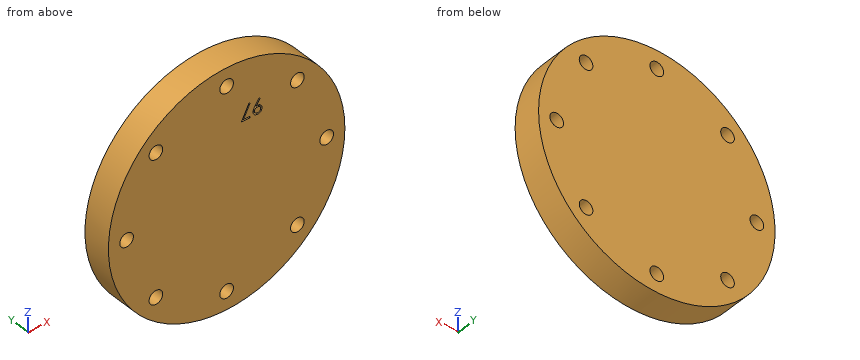
from build123d import *

# Parameters (mm, degrees)
SKETCH1_R           = 26
BOSS_EXTRUDE1_DEPTH = 6.2
SKETCH4_R           = 1.5
CUT_EXTRUDE1_DEPTH  = 13
SKETCH5_R           = 1.5
CUT_EXTRUDE2_DEPTH  = 10
CUT_EXTRUDE3_DEPTH  = 1


with BuildPart() as part:
    # Sketch1 → Boss-Extrude1 (new body)
    with BuildSketch(Plane(origin=(0, 0, 0), x_dir=(1, 0, 0), z_dir=(0, 1, 0))):
        Circle(SKETCH1_R)
    extrude(amount=BOSS_EXTRUDE1_DEPTH)

    # Sketch4 → Cut-Extrude1 (cut)
    with BuildSketch(Plane.XZ):
        with Locations((22, 0)):
            Circle(SKETCH4_R)
    extrude(amount=-CUT_EXTRUDE1_DEPTH, mode=Mode.SUBTRACT)

    # Sketch5 → Cut-Extrude2 (cut)
    with BuildSketch(Plane.XZ):
        with Locations((-22, 0)):
            Circle(SKETCH5_R)
        with Locations((0, 22)):
            Circle(SKETCH5_R)
        with Locations((0, -22)):
            Circle(SKETCH5_R)
        with Locations((-15.556349186, 15.556349186)):
            Circle(SKETCH5_R)
        with Locations((15.556349186, 15.556349186)):
            Circle(SKETCH5_R)
        with Locations((15.556349186, -15.556349186)):
            Circle(SKETCH5_R)
        with Locations((-15.556349186, -15.556349186)):
            Circle(SKETCH5_R)
    extrude(amount=-CUT_EXTRUDE2_DEPTH, mode=Mode.SUBTRACT)

    # Sketch6 → Cut-Extrude3 (cut)
    with BuildSketch(Plane(origin=(0, 0, 0), x_dir=(-1, 0, 0), z_dir=(0, -1, 0))):
        with BuildLine():
            Line((-7.133469585, -15.941578498), (-7.361163896, -15.783210108))
            Line((-7.361163896, -15.783210108), (-6.478371428, -14.492730341))
            add(Edge.make_bspline(
                [(-6.478371428, -14.492730341), (-6.534696595, -14.499618334), (-6.64560399, -14.513181177), (-6.757306933, -14.515672785), (-6.812280683, -14.516899011)],
                knots=[0, 0, 0, 0, 0.000170115, 0.000334967, 0.000334967, 0.000334967, 0.000334967], degree=3))
            add(Edge.make_bspline(
                [(-6.812280683, -14.516899011), (-6.845610969, -14.51604532), (-6.911035406, -14.5143696), (-7.007221263, -14.501087388), (-7.099646021, -14.4806312), (-7.188064651, -14.450106973), (-7.272809488, -14.412171883), (-7.353695528, -14.365130163), (-7.430613885, -14.309788742), (-7.502738465, -14.246440242), (-7.568335542, -14.176882295), (-7.626776676, -14.103262533), (-7.675346132, -14.02472576), (-7.715692748, -13.94287406), (-7.746291089, -13.856530978), (-7.768572819, -13.766679022), (-7.782290955, -13.672688461), (-7.783922991, -13.608712092), (-7.784751636, -13.576228939)],
                knots=[0, 0, 0, 0, 9.9954e-05, 0.000196201, 0.000290782, 0.000383503, 0.000476303, 0.000568919, 0.000663705, 0.000760153, 0.000856434, 0.000950205, 0.001041624, 0.001132931, 0.001223461, 0.001315861, 0.001410305, 0.001507717, 0.001507717, 0.001507717, 0.001507717], degree=3))
            add(Edge.make_bspline(
                [(-7.784751636, -13.576228939), (-7.783178256, -13.531807375), (-7.78009003, -13.444616857), (-7.755235661, -13.317223367), (-7.714359496, -13.196767002), (-7.657365183, -13.083564469), (-7.585578686, -12.979244184), (-7.499301608, -12.885256374), (-7.399058726, -12.802937828), (-7.287133608, -12.732176987), (-7.166163368, -12.675267382), (-7.039463942, -12.633321731), (-6.908006134, -12.608648581), (-6.818954033, -12.605395693), (-6.774119625, -12.603757985)],
                knots=[0, 0, 0, 0, 0.000133185, 0.000261414, 0.000387724, 0.00051373, 0.000640399, 0.00076644, 0.000895188, 0.001028407, 0.001162697, 0.001295241, 0.001427846, 0.0015623, 0.0015623, 0.0015623, 0.0015623], degree=3))
            add(Edge.make_bspline(
                [(-6.774119625, -12.603757985), (-6.730133702, -12.605418204), (-6.643221663, -12.608698641), (-6.515415207, -12.632723385), (-6.393004427, -12.673215224), (-6.276667904, -12.729171935), (-6.168954294, -12.799313044), (-6.072093379, -12.882892219), (-5.988295569, -12.979961519), (-5.917698191, -13.088173221), (-5.861028941, -13.204438982), (-5.820141941, -13.325800112), (-5.794972683, -13.451383809), (-5.791801015, -13.536468796), (-5.790200354, -13.579409027)],
                knots=[0, 0, 0, 0, 0.000131915, 0.000260652, 0.000388569, 0.000517718, 0.000646848, 0.000773094, 0.000900237, 0.001030248, 0.001159674, 0.001287189, 0.001413545, 0.001542287, 0.001542287, 0.001542287, 0.001542287], degree=3))
            add(Edge.make_bspline(
                [(-5.790200354, -13.579409027), (-5.79126934, -13.612740873), (-5.793437509, -13.680346185), (-5.80861973, -13.783062281), (-5.834400898, -13.887793039), (-5.863657796, -13.976440487), (-5.89189912, -14.049654581), (-5.918479432, -14.107486371), (-5.9479726, -14.168356803), (-5.982370337, -14.231627602), (-6.019347564, -14.29810533), (-6.061129907, -14.367123223), (-6.106764248, -14.438773895), (-6.139266922, -14.48707661), (-6.155910491, -14.51181087)],
                knots=[0, 0, 0, 0, 9.9984e-05, 0.000202793, 0.000310776, 0.000423207, 0.000482616, 0.000546097, 0.000614079, 0.0006855, 0.000762103, 0.000842274, 0.000927493, 0.001016928, 0.001016928, 0.001016928, 0.001016928], degree=3))
            Line((-6.155910491, -14.51181087), (-7.133469585, -15.941578498))
        make_face()
        with BuildLine():
            add(Edge.make_bspline(
                [(-6.75949122, -14.191257985), (-6.734241793, -14.190568208), (-6.685089742, -14.189225448), (-6.613083192, -14.181052778), (-6.545116236, -14.166562091), (-6.481007317, -14.145770638), (-6.420113628, -14.120682088), (-6.363402387, -14.088739786), (-6.310826133, -14.050624696), (-6.262032799, -14.007798468), (-6.218704028, -13.960218295), (-6.180111422, -13.910418777), (-6.147308621, -13.85818131), (-6.121397648, -13.802851707), (-6.100093783, -13.745776811), (-6.08538173, -13.686037503), (-6.077231656, -13.623945025), (-6.075842299, -13.5817641), (-6.075136252, -13.560328498)],
                knots=[0, 0, 0, 0, 7.5753e-05, 0.000147465, 0.000217073, 0.000283852, 0.000349411, 0.000414338, 0.000478589, 0.000543925, 0.000608743, 0.000671332, 0.000732749, 0.000793345, 0.000854313, 0.000915245, 0.00097749, 0.001041807, 0.001041807, 0.001041807, 0.001041807], degree=3))
            add(Edge.make_bspline(
                [(-6.075136252, -13.560328498), (-6.075743737, -13.538883944), (-6.076940862, -13.496624821), (-6.086545056, -13.434440415), (-6.103440794, -13.374847242), (-6.126110733, -13.317519052), (-6.155974092, -13.262926858), (-6.191809397, -13.21038526), (-6.234383834, -13.160227401), (-6.283371876, -13.11363293), (-6.336198935, -13.070681622), (-6.392496674, -13.032775681), (-6.451801062, -13.001006453), (-6.513750292, -12.974790959), (-6.578473437, -12.954333277), (-6.645932198, -12.93962181), (-6.716467459, -12.931483147), (-6.764347626, -12.930102571), (-6.788748031, -12.929399011)],
                knots=[0, 0, 0, 0, 6.4316e-05, 0.000126743, 0.000188161, 0.000249812, 0.000311283, 0.000374438, 0.00044032, 0.000508243, 0.00057698, 0.000644365, 0.000711521, 0.0007785, 0.000845884, 0.000914871, 0.00098532, 0.001058531, 0.001058531, 0.001058531, 0.001058531], degree=3))
            add(Edge.make_bspline(
                [(-6.788748031, -12.929399011), (-6.812936227, -12.930103708), (-6.860393269, -12.931486318), (-6.930301471, -12.93960634), (-6.997304101, -12.954432215), (-7.061839714, -12.974781483), (-7.123787103, -13.001008409), (-7.183088694, -13.032777346), (-7.239399603, -13.070672896), (-7.292176014, -13.113666725), (-7.341250557, -13.160010519), (-7.383093001, -13.210604986), (-7.419010318, -13.262899526), (-7.448832642, -13.317526316), (-7.471513497, -13.374845304), (-7.488406312, -13.43444094), (-7.498011291, -13.496624685), (-7.499208308, -13.538883898), (-7.499815739, -13.560328498)],
                knots=[0, 0, 0, 0, 7.2576e-05, 0.000142393, 0.000210758, 0.000278143, 0.000345121, 0.000412278, 0.000479663, 0.0005484, 0.000616323, 0.000681795, 0.00074495, 0.000806421, 0.000868072, 0.00092949, 0.000991917, 0.001056233, 0.001056233, 0.001056233, 0.001056233], degree=3))
            add(Edge.make_bspline(
                [(-7.499815739, -13.560328498), (-7.499266077, -13.581780792), (-7.498182044, -13.624088644), (-7.487724692, -13.686251872), (-7.470236538, -13.745840447), (-7.446814663, -13.803433775), (-7.415970363, -13.858471817), (-7.378120872, -13.910693638), (-7.333756556, -13.960691225), (-7.283470463, -14.007687768), (-7.228435774, -14.050824384), (-7.169655869, -14.088498373), (-7.10814266, -14.120314091), (-7.043679609, -14.145842346), (-6.97674444, -14.166354355), (-6.906735571, -14.181026071), (-6.833884527, -14.189147056), (-6.784526901, -14.190547591), (-6.75949122, -14.191257985)],
                knots=[0, 0, 0, 0, 6.4316e-05, 0.000126844, 0.000188436, 0.000250326, 0.000312966, 0.000377217, 0.000443451, 0.000513196, 0.000583426, 0.000652939, 0.000722346, 0.000790847, 0.000860662, 0.000932137, 0.001005113, 0.00108023, 0.00108023, 0.00108023, 0.00108023], degree=3))
        make_face(mode=Mode.SUBTRACT)
        Polygon((-5.179623431, -12.685168241), (-3.225777277, -12.685168241), (-4.894687534, -15.941578498), (-5.140826356, -15.806106743), (-3.70787864, -13.010809267), (-5.179623431, -13.010809267), align=None)
    extrude(amount=-CUT_EXTRUDE3_DEPTH, mode=Mode.SUBTRACT)


solid = part.part
Geometry check sheet. Reference: the model listing, model coordinates, mm. Give positions to 0.01 mm unless a question says otherwise; leave off trailing zeros. Loops run counter-clockwise (first coordinate to the right, second up) from the corner with the lowest first, then second, coordinate; pieces in that order, holes last. Notation, with made-up numbers: (73, -24.5) -> (105, -24.5) arc R17 cw to (105, 7.5) -> close; hole circle Ø8 at (10, 66.5). An arc over 180 degrees is marked (long way). Answer in a Markdown table with one row per item. Add a question column.
1) Material ranges on probe 1 along Z at (x, y) = (0, 4.75); probe 2 along Z at (x, y) = (-15, 3.5); probe 3 along X at (y, z) = (6, -16), recorded low to high. Write a range as from..to.
2) Cross-section at C-C on z = -22. Record the boundary of the cut face in (x, y).
3) Cross-section at A-A on z = 0. Record the boundary of the cut face in (x, y).
4) Gauge pin test, flat ends, axial feed: P1, Ø0.8, axis at x = 4.5, y = 0.5, coming from the -Z side; P2, Ø2.5, axis at x = -15.56, z = -15.56, coming from the -Y side; P3, Ø1.5, axis at x = 8, z = -17, coming from the -Y side; P4, Ø1.5, axis at x = 19, y = 4, coming from the -Z side. Record the tip position at first contact, or that the pin passes through.
5) Cross-section at B-B on x = 0. Record the boundary of the cut face in (y, z), and give its area (3 significant figures).
6) Cross-section at D-D on x = 22. Record the boundary of the cut face in (y, z).
Outcome:
| question | item | result |
|---|---|---|
| 1 | probe 1 | z = -26..-23.5, -20.5..20.5, 23.5..26 |
| 1 | probe 2 | z = -21.24..-16.95, -14.16..14.16, 16.95..21.24 |
| 1 | probe 3 | x = -20.49..-16.99, -14.12..14.12, 16.99..20.49 |
| 2 | outline | (-13.86, 0) -> (-1.5, 0) -> (-1.5, 6.2) -> (-13.86, 6.2) -> close; (1.5, 0) -> (13.86, 0) -> (13.86, 6.2) -> (1.5, 6.2) -> close |
| 3 | outline | (-26, 0) -> (-23.5, 0) -> (-23.5, 6.2) -> (-26, 6.2) -> close; (-20.5, 0) -> (20.5, 0) -> (20.5, 6.2) -> (-20.5, 6.2) -> close; (23.5, 0) -> (26, 0) -> (26, 6.2) -> (23.5, 6.2) -> close |
| 4 | P1 | stops at z = -25.67 |
| 4 | P2 | passes through |
| 4 | P3 | stops at y = 0 |
| 4 | P4 | stops at z = -18.52 |
| 5 | outline | (0, -26) -> (6.2, -26) -> (6.2, -23.5) -> (0, -23.5) -> close; (0, -20.5) -> (6.2, -20.5) -> (6.2, 20.5) -> (0, 20.5) -> close; (0, 23.5) -> (6.2, 23.5) -> (6.2, 26) -> (0, 26) -> close |
| 5 | area | 285 mm^2 |
| 6 | outline | (0, -13.86) -> (6.2, -13.86) -> (6.2, -1.5) -> (0, -1.5) -> close; (0, 1.5) -> (6.2, 1.5) -> (6.2, 13.86) -> (0, 13.86) -> close |
